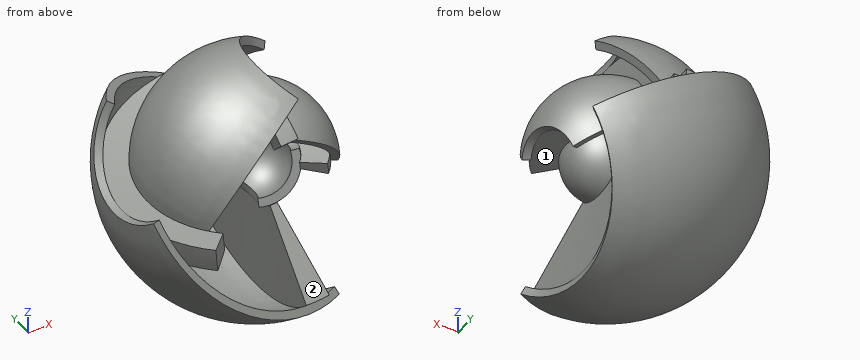
```python
from build123d import *

# Parameters (mm, degrees)
SWEEP2_ANGLE = 135


# Read off the part's stored shape, not the designer's step: Sweep2
with BuildPart() as part:
    # Sweep2 outline → Sweep2 (revolve)
    with BuildSketch(Plane(origin=(0, 0, 0), x_dir=(0.5416752204196997, -0.707106781186551, -0.4545194776720406), z_dir=(-0.5416752204197053, -0.7071067811865439, 0.4545194776720451))):
        with BuildLine():
            Line((32.139380484, -38.302222156), (39.852831801, -47.494755473))
            ThreePointArc((39.852831801, -47.494755473), (62, 0), (39.852831801, 47.494755473))
            Line((39.852831801, 47.494755473), (32.139380484, 38.302222156))
            ThreePointArc((32.139380484, 38.302222156), (50, 0), (32.139380484, -38.302222156))
        make_face()
    revolve(axis=Axis((0, 0, 0), (0.6427876096865381, 0, 0.7660444431189789)), revolution_arc=SWEEP2_ANGLE)



with BuildPart() as body_2:
    # Sweep3: sweep along a path in Sketch15
    with BuildLine(Plane(origin=(0, 0, 0), x_dir=(-0.49999999999999506, 0, -0.8660254037844415), z_dir=(0.8660254037844415, 0, -0.49999999999999506))) as sweep3_path:
        ThreePointArc((0, 106.00000000000001), (-97.93123044619651, 40.56444383069927), (-74.95331880577362, -74.95331880577444))
    # Sketch2 → Sweep3 (sweep)
    with BuildSketch(Plane(origin=(0, 0, 0), x_dir=(1, 0, 0), z_dir=(0, 1, 0))):
        with BuildLine():
            Line((100, -3.4668e-13), (112, -3.9105e-13))
            ThreePointArc((112, -3.9105e-13), (71.99221228489193, -85.79697762932594), (-19.448595898696997, -110.29846833736717))
            Line((-19.448595898696997, -110.29846833736717), (-17.364817766693747, -98.48077530122067))
            ThreePointArc((-17.364817766693747, -98.48077530122067), (64.27876096865351, -76.60444431189816), (100, -3.4668e-13))
        make_face()
    sweep(path=sweep3_path.line)


with BuildPart() as body_3:
    # Sweep4: sweep along a path in Sketch16
    with BuildLine(Plane(origin=(0, 0, 0), x_dir=(0.7660444431189743, 0, -0.6427876096865438), z_dir=(0.6427876096865438, 0, 0.7660444431189745))) as sweep4_path:
        ThreePointArc((0, 156), (-144.12520707176088, 59.69861544895363), (-110.3086578651008, -110.308657865102))
    # Sketch3 → Sweep4 (sweep)
    with BuildSketch(Plane(origin=(0, 0, 0), x_dir=(1, 0, 0), z_dir=(0, 1, 0))):
        with BuildLine():
            Line((-1.04744e-12, -150), (-1.13124e-12, -162))
            ThreePointArc((-1.13124e-12, -162), (-124.09919978527539, -104.13159276921829), (-159.53885598797743, 28.13100478204443))
            Line((-159.53885598797743, 28.13100478204443), (-147.72116295183096, 26.047226650041136))
            ThreePointArc((-147.72116295183096, 26.047226650041136), (-114.90666646784759, -96.4181414529799), (-1.04744e-12, -150))
        make_face()
    sweep(path=sweep4_path.line)


with BuildPart() as body_4:
    # Sweep5: sweep along a path in Sketch17
    with BuildLine(Plane(origin=(0, 0, 0), x_dir=(0.5000000000000013, 0, 0.8660254037844379), z_dir=(-0.8660254037844378, 0, 0.5000000000000012))) as sweep5_path:
        ThreePointArc((0, 206.00000000000003), (-190.3191836973253, 78.83278706720802), (-145.663996924428, -145.66399692442957))
    # Sketch4 → Sweep5 (sweep)
    with BuildSketch(Plane(origin=(0, 0, 0), x_dir=(1, 0, 0), z_dir=(0, 1, 0))):
        with BuildLine():
            Line((-200, -7.4728e-13), (-212, -7.9212e-13))
            ThreePointArc((-212, -7.9212e-13), (-136.27097325354666, 162.40142194122313), (36.81341366538924, 208.77924363858813))
            Line((36.81341366538924, 208.77924363858813), (34.72963553338607, 196.9615506024416))
            ThreePointArc((34.72963553338607, 196.9615506024416), (-128.55752193730814, 153.2088886237954), (-200, -7.4728e-13))
        make_face()
    sweep(path=sweep5_path.line)


with BuildPart() as part_1:
    add(part.part)

    add(body_2.part)  # Sweep6 merges body 2
    # Sweep6: sweep along a path in Sketch22
    with BuildLine(Plane(origin=(0, 0, 0), x_dir=(-0.9961946980917453, 0, -0.08715574274766177), z_dir=(0.08715574274766177, 0, -0.9961946980917453))) as sweep6_path:
        ThreePointArc((0, 77.99999999999999), (-72.06260353588043, 29.849307724476812), (-55.1543289325504, -55.154328932551))
    # Sketch5 → Sweep6 (sweep)
    with BuildSketch(Plane(origin=(0, 0, 0), x_dir=(1, 0, 0), z_dir=(0, 1, 0))):
        with BuildLine():
            Line((62, -2.1647e-13), (100, -3.4915e-13))
            ThreePointArc((100, -3.4915e-13), (99.61946980917453, -8.715574274766185), (98.48077530122076, -17.364817766693417))
            Line((98.48077530122076, -17.364817766693417), (61.058080686756846, -10.766187015349916))
            ThreePointArc((61.058080686756846, -10.766187015349916), (61.76407128168819, -5.403656050355033), (62, -2.1647e-13))
        make_face()
    sweep(path=sweep6_path.line)


with BuildPart() as sweep7_tool:
    # Sweep7: sweep along a path in Sketch23
    with BuildLine(Plane(origin=(0, 0, 0), x_dir=(0.08715574274765134, 0, -0.9961946980917462), z_dir=(0.9961946980917462, 0, 0.08715574274765134))) as sweep7_path:
        ThreePointArc((0, 128), (-118.25658016144483, 48.98347934273119), (-90.50966799187758, -90.50966799187859))
    # Sketch6 → Sweep7 (sweep)
    with BuildSketch(Plane(origin=(0, 0, 0), x_dir=(1, 0, 0), z_dir=(0, 1, 0))):
        with BuildLine():
            Line((-3.86585e-12, -112), (-5.17747e-12, -150))
            ThreePointArc((-5.17747e-12, -150), (-13.073361412153913, -149.4292047137614), (-26.047226650044717, -147.72116295183034))
            Line((-26.047226650044717, -147.72116295183034), (-19.448595898700052, -110.29846833736664))
            ThreePointArc((-19.448595898700052, -110.29846833736664), (-9.761443187741587, -111.57380618627518), (-3.86585e-12, -112))
        make_face()
    sweep(path=sweep7_path.line)


with BuildPart() as part_2:
    add(part_1.part)


with BuildPart() as part_3:
    # Sweep7: joined with sweep7_tool
    add(part_2.part.fuse(sweep7_tool.part, body_3.part, tol=0.00001))


    add(body_4.part)  # Sweep8 merges body 4
    # Sweep8: sweep along a path in Sketch24
    with BuildLine(Plane(origin=(0, 0, 0), x_dir=(0.9961946980917459, 0, 0.08715574274765439), z_dir=(-0.08715574274765439, 0, 0.996194698091746))) as sweep8_path:
        ThreePointArc((0, 178), (-164.45055678700922, 68.11765096098556), (-125.86500705120477, -125.86500705120612))
    # Sketch7 → Sweep8 (sweep)
    with BuildSketch(Plane(origin=(0, 0, 0), x_dir=(1, 0, 0), z_dir=(0, 1, 0))):
        with BuildLine():
            Line((-162, -6.053e-13), (-200, -7.4728e-13))
            ThreePointArc((-200, -7.4728e-13), (-199.23893961834912, 17.431148549531017), (-196.9615506024417, 34.72963553338542))
            Line((-196.9615506024417, 34.72963553338542), (-159.53885598797785, 28.131004782042204))
            ThreePointArc((-159.53885598797785, 28.131004782042204), (-161.38354109086288, 14.119230325120132), (-162, -6.053e-13))
        make_face()
    sweep(path=sweep8_path.line)

    # Sweep9: sweep along a path in Sketch25
    with BuildLine(Plane(origin=(0, 0, 0), x_dir=(-0.08715574274765836, 0, 0.9961946980917455), z_dir=(-0.9961946980917457, 0, -0.08715574274765837))) as sweep9_path:
        ThreePointArc((0, 128), (-118.25658016144483, 48.98347934273119), (-90.50966799187758, -90.50966799187859))
    # Sketch8 → Sweep9 (sweep)
    with BuildSketch(Plane(origin=(0, 0, 0), x_dir=(1, 0, 0), z_dir=(0, 1, 0))):
        with BuildLine():
            Line((10.766187015349702, 61.05808068675688), (34.72963553338614, 196.96155060244158))
            ThreePointArc((34.72963553338614, 196.96155060244158), (17.43114854953167, 199.2389396183491), (0, 200))
            Line((0, 200), (0, 61.99999999999999))
            ThreePointArc((0, 61.99999999999999), (5.403656050354817, 61.76407128168821), (10.766187015349702, 61.05808068675688))
        make_face()
    sweep(path=sweep9_path.line)


solid = part_3.part
```
Geometry: final body of the model. Coordinates: model frame, mm. Face numbers are marked on the shaded views. A direction names the side the tool comes from. Round coordinates to 2 decimals unless told otherwise and drop trailing zeros.
Item 1: Set-up query: the marked faces 1 and 2. Return all of +Z, -Z, +X, -X, +Y, -Y with unobstructed straight access to the full face (end or side cutting, diameter ignored); none if empty.
Item 2: Pin query (flat end, axial travel): P1, Ø12, axis at y = -38.5, z = -126, coming from the +X side; P2, Ø8, axis at x = -76, y = 110.5, coming from the +Z side; P3, Ø12, axis at x = -175.5, y = 31, coming from the -Z side. Return the tip coordinate at first contact, or that it passes through.
Item 3: Material intervals for L1, parallel to X at y = 36.5, z = 23; L2, parallel to X at y = 119.5, z = -42; L3, parallel to Y at x = -111.5, z = 42.5, sorted ascending.
Completed:
1. face 1: none
1. face 2: -Y
2. P1: stops at x = 23.77
2. P2: stops at z = 96.51
2. P3: stops at z = -123.63
3. L1: x = -156.15 to -143.66, 25.27 to 44.53, 90.22 to 103.36
3. L2: x = -170 to -154.78, -100.99 to -80.35, -7.43 to 14.83
3. L3: y = -109.57 to -90.89, 90.89 to 109.57, 160.5 to 175.23
